For this review, take the finished solid that the model builds, in its own axes (mm). A direction names the side the tool comes from. Round coordinates to 2 decimals unless told otherwise and drop trailing zeros. Order: outer loops, then holes, each group sorted by start corner. A loop starts at its lowest first (then second) coordinate and runs counter-clockwise, first axis right, second up. Notation, with made-up numbers: (89, -7.5) -> (134, -7.5) arc R7 ccw to (134, -2.5) -> close; hole circle Ø9 at (-27.5, 40.25). An arc over 180 degrees is marked (long way). Answer in a Markdown table with one row per item.
```python
from build123d import *

# Parameters (mm, degrees)
SKETCH1_R           = 7.7
SKETCH1_R_2         = 4
BOSS_EXTRUDE1_DEPTH = 4
SKETCH2_R           = 6
CUT_EXTRUDE1_DEPTH  = 2.8
SKETCH3_R           = 1.15
CUT_EXTRUDE2_DEPTH  = 12.600862037


with BuildPart() as part:
    # Sketch1 → Boss-Extrude1 (new body)
    with BuildSketch(Plane(origin=(0, 0, 0), x_dir=(1, 0, 0), z_dir=(0, 1, 0))):
        with Locations(Location((0, 0, 0), (0, 0, 270))):
            Circle(SKETCH1_R)
        with Locations(Location((0, 0, 0), (0, 0, 270))):
            Circle(SKETCH1_R_2, mode=Mode.SUBTRACT)
    extrude(amount=BOSS_EXTRUDE1_DEPTH)

    # Sketch2 → Cut-Extrude1 (cut)
    with BuildSketch(Plane.XZ):
        with Locations(Location((0, 0, 0), (0, 0, 270))):
            Circle(SKETCH2_R)
    extrude(amount=-CUT_EXTRUDE1_DEPTH, mode=Mode.SUBTRACT)

    # Sketch3 → Cut-Extrude2 (cut, through all)
    with BuildSketch(Plane(origin=(0, 4, 0), x_dir=(1, 0, 0), z_dir=(0, 1, 0))):
        with Locations((4.772970773, 4.772970773)):
            Circle(SKETCH3_R)
        with Locations((-4.772970773, -4.772970773)):
            Circle(SKETCH3_R)
    extrude(amount=-CUT_EXTRUDE2_DEPTH, mode=Mode.SUBTRACT)


solid = part.part
```
Q1. Take a section at C-C, the plane y = 1.1. Write out the cut boundary in (x, z).
Answer key:
| item | result |
|---|---|
| outline | (-5.91, 4.93) arc R7.7 ccw to (4.93, -5.91) arc R1.15 cw to (3.62, -4.78) arc R6 cw to (-4.78, 3.62) arc R1.15 cw to start; (-4.93, 5.91) arc R1.15 cw to (-3.62, 4.78) arc R6 cw to (4.78, -3.62) arc R1.15 cw to (5.91, -4.93) arc R7.7 ccw to start |
Q2. Clearance check with flat-ended pins moving along their axes: pin 1 Ø1 at (y, z) = (2.5, -1.5) entering from +X; pin 2 Ø3 at (x, z) = (-1.5, -3.5) entering from -Y; pin 3 Ø1.5 at (x, y) = (1.5, 1) entering from +Z. State where each tip first meets the part, or that it passes through.
Answer key:
| item | result |
|---|---|
| pin 1 | stops at x = 7.63 |
| pin 2 | stops at y = 2.8 |
| pin 3 | stops at z = 7.66 |
Q3. To check wall thickness, follow probe 1 along Z at (x, y) = (0, 3.25); probe 2 along Y at (x, z) = (-2.5, -3.25); probe 3 along X at (y, z) = (1.2, 0). State the ranges of each line that lie inside material, in increasing order.
Answer key:
| item | result |
|---|---|
| probe 1 | z = -7.7 to -4, 4 to 7.7 |
| probe 2 | y = 2.8 to 4 |
| probe 3 | x = -7.7 to -6, 6 to 7.7 |
Q4. Take a section at A-A, the plane z = 0. Write out the cut boundary in (x, y).
Answer key:
| item | result |
|---|---|
| outline | (-7.7, 0) -> (-6, 0) -> (-6, 2.8) -> (-4, 2.8) -> (-4, 4) -> (-7.7, 4) -> close; (4, 2.8) -> (6, 2.8) -> (6, 0) -> (7.7, 0) -> (7.7, 4) -> (4, 4) -> close |
Q5. The part is to be moulded in two halves that separate along X. For faces 1 (the face through (-3.696, 2.028, 5.177)), 2 (the face through (-3.905, 3.392, -0.867)), 3 (the face through (-5.331, 1.972, -5.556)), 4 (the face through (-3, 4, 3)), say which applies: +X half, -X half, draft (parallel to the pull), parting line (faces both ways), or undercut.
Answer key:
| item | result |
|---|---|
| face 1 | undercut |
| face 2 | undercut |
| face 3 | parting line |
| face 4 | draft |
Q6. Tool access review of faces 5 (the face through (5.331, 1.972, 5.556)), 6 (the face through (-4.327, 1.38, -4.157)): name each direction out of +Z, -Z, +X, -X, +Y, -Y from which nothing blocks a thin tool from reaching the whole face with its end or side.
Answer key:
| item | result |
|---|---|
| face 5 | +Y, -Y |
| face 6 | -Y |
Q7. Take a section at B-B, the plane x = -2. Write out the cut boundary in (y, z), then the cut area to 3 significant figures.
Answer key:
| item | result |
|---|---|
| outline | (0, -7.44) -> (4, -7.44) -> (4, -3.46) -> (2.8, -3.46) -> (2.8, -5.66) -> (0, -5.66) -> close; (0, 5.66) -> (2.8, 5.66) -> (2.8, 3.46) -> (4, 3.46) -> (4, 7.44) -> (0, 7.44) -> close |
| area | 19.5 mm^2 |
Q8. Take a section at D-D, the plane x = 4.25. Write out the cut boundary in (y, z).
Answer key:
| item | result |
|---|---|
| outline | (0, -6.42) -> (4, -6.42) -> (4, -5.8) -> (0, -5.8) -> close; (0, 4.24) -> (2.8, 4.24) -> (2.8, -3.75) -> (4, -3.75) -> (4, 6.42) -> (0, 6.42) -> close |
